from build123d import *

# Parameters (mm, degrees)
SKETCH6_R           = 3.687499751
CUT_EXTRUDE3_DEPTH  = 29.1338
SKETCH7_R           = 2.413
BOSS_EXTRUDE1_DEPTH = 16.51
SKETCH9_R           = 4.699
CUT_EXTRUDE4_DEPTH  = 6.35
SKETCH10_W          = 6.35
SKETCH10_H          = 6.35
BOSS_EXTRUDE3_DEPTH = 3.81


with BuildPart() as part:
    # Sketch1 → Revolve1 (revolve)
    with BuildSketch(Plane(origin=(0, 0, 0), x_dir=(0, 0, -1), z_dir=(1, 0, 0))):
        Polygon((4.892085627, 0), (44.3738, 0), (44.3738, 2.159), (43.409235, 3.123565), (25.3238, 3.123565), (18.9738, 3.133725), (6.4516, 3.133725), (6.2738, 3.133725), (6.2738, 3.311525), (6.2738, 4.445), (6.2738, 4.699), (6.0198, 4.699), (0.635, 4.699), (0, 4.699), (0, 4.064), (0, 3.19405), (0, 0), align=None)
    revolve(axis=Axis((0, 0, -4.892085627), (0, 0, -1)))

    # Sketch6 → Cut-Extrude3 (cut)
    with BuildSketch(Plane(origin=(0, 0, -44.3738), x_dir=(-1, 0, 0), z_dir=(0, 0, -1))):
        Circle(SKETCH6_R)
    extrude(amount=-CUT_EXTRUDE3_DEPTH, mode=Mode.SUBTRACT)

    # Sketch7 → Boss-Extrude1 (add)
    with BuildSketch(Plane(origin=(0, 0, -15.24), x_dir=(-1, 0, 0), z_dir=(0, 0, -1))):
        Circle(SKETCH7_R)
    extrude(amount=BOSS_EXTRUDE1_DEPTH)

    # Sketch9 → Cut-Extrude4 (cut)
    with BuildSketch(Plane.XY):
        Circle(SKETCH9_R)
    extrude(amount=-CUT_EXTRUDE4_DEPTH, mode=Mode.SUBTRACT)

    # Sketch10 → Boss-Extrude3 (add)
    with BuildSketch(Plane.XY.offset(-6.35)):
        Rectangle(SKETCH10_W, SKETCH10_H)
    extrude(amount=BOSS_EXTRUDE3_DEPTH)


solid = part.part
The listing builds one solid part. Answer for the finished solid, in the listing's coordinates (mm). A direction names the side the tool comes from. Give positions to 0.01 mm unless a question says otherwise; leave off trailing zeros. Loops run counter-clockwise (first coordinate to the right, second up) from the corner with the lowest first, then second, coordinate; pieces in that order, holes last. Notation, with made-up numbers: (-0.75, 21) - (54.25, 21) arc R13 ccw to (54.25, 43) - close; hole circle Ø9 at (-34, -10.75). An arc over 180 degrees is marked (long way). Answer as a JSON object with one key per item and string values.
1. A cutting plane is placed at D-D (z = -12). Write down the section's boundary in (x, y), then the cut area to 3 significant figures.
Determined:
{"outline": "circle Ø6.27 at (0, 0)", "area": "30.9 mm²"}
2. Find the intervals of material crossed by L1, parallel to Y at x = 2, z = -7.5; L2, parallel to Z at x = -2.25, y = -2, in increasing order. Write a range as [from, to].
Determined:
{"L1": "[-2.41, 2.41]", "L2": "[-15.24, -2.54]"}
3. Flat-ended cylindrical pins translate along their axes: pin 1 Ø1.5 at (y, z) = (2, -19) entering from +X; pin 2 Ø3 at (x, z) = (1.5, -21) entering from -Y. Find the tip coordinate at first contact, or state that the pin passes through.
Determined:
{"pin 1": "x = 2.06", "pin 2": "y = -2.41"}
4. A cutting plane is placed at A-A (x = 0). Write down the section's boundary in (y, z) (3 decimals), then the cut area to 3 significant figures.
Determined:
{"outline": "(-3.175, -6.35) - (-3.134, -6.35) - (-3.134, -15.24) - (-2.413, -15.24) - (-2.413, -31.75) - (2.413, -31.75) - (2.413, -15.24) - (3.134, -15.24) - (3.134, -6.35) - (3.175, -6.35) - (3.175, -2.54) - (-3.175, -2.54) - close", "area": "160 mm²"}
5. A cutting plane is placed at C-C (z = -20). Write down the section's boundary in (x, y).
Determined:
{"outline": "circle Ø4.83 at (0, 0)"}
6. For faces 1 (the flat face through (0, 0, -31.75)), 2 (the cylindrical face through (-3.06, -0.68, -10.73)), determine the directions among +Z, -Z, +X, -X, +Y, -Y from which every point of the face is accessible in a straight line to the end or side of a thin tool.
Determined:
{"face 1": "-Z, +X, -X, +Y, -Y", "face 2": "-Z"}
7. A cutting plane is placed at B-B (y = 2). Write down the section's boundary in (x, z) (3 decimals), then the cut area to 3 significant figures.
Determined:
{"outline": "(-3.175, -6.35) - (-2.413, -6.35) - (-2.413, -15.24) - (-1.35, -15.24) - (-1.35, -31.75) - (1.35, -31.75) - (1.35, -15.24) - (2.413, -15.24) - (2.413, -6.35) - (3.175, -6.35) - (3.175, -2.54) - (-3.175, -2.54) - close", "area": "112 mm²"}
